Answer from the drawing. Dimensions are ordinates in mm from the lowest x, y and z of the part. A direction names the side the tool comes from. Coordinates: 2 decimals unless noted, no trailing zeros. Write each loop counter-clockwise with the first axis right and the second up, starting at its lowest first coordinate (ties: lowest second). Pieces come first, ordered by that corner, then holes. Notation, with made-up numbers: (31, -20) -> (86, -20) arc R10 ccw to (86, -12) -> close; hole circle Ø4 at (44.25, 73). An arc over 180 degrees is marked (long way). One line per item, written item: value. Start each with the question number.
1. Consider line 1 along Y through (x, z) = (15, 23.75); line 2 along X through (y, z) = (2.5, 14.5); line 3 along Y through (x, z) = (19, 14.25). Determine where each line is inside the solid, lowest interval first.
2. Given P1, Ø3, axis at x = 4.5, y = 7.5, coming from the +Z side; P2, Ø12, axis at y = 3, z = 9, coming from the +X side; P3, Ø3, axis at x = 20, y = 6.5, coming from the +Z side; P4, Ø3, axis at y = 18, z = 13.5, coming from the +X side, each flat-ended and moving along its own axis, determine where each tip first touches the part or whether it passes through.
3. Find section D-D, the plane y = 16.25. Write down the section's boundary in (x, z).
4. For the marked faces 1, 2 and 3, determine the directions among +Z, -Z, +X, -X, +Y, -Y from which every point of the face is accessible in a straight line to the end or side of a thin tool.
5. Find section C-C, the plane y = 4.25. Write down the section's boundary in (x, z), and give its area (3 significant figures).
6. Find section A-A, the plane z = 15. Write down the section's boundary in (x, y).
7. Find section B-B, the plane x = 15. Write down the section's boundary in (y, z).
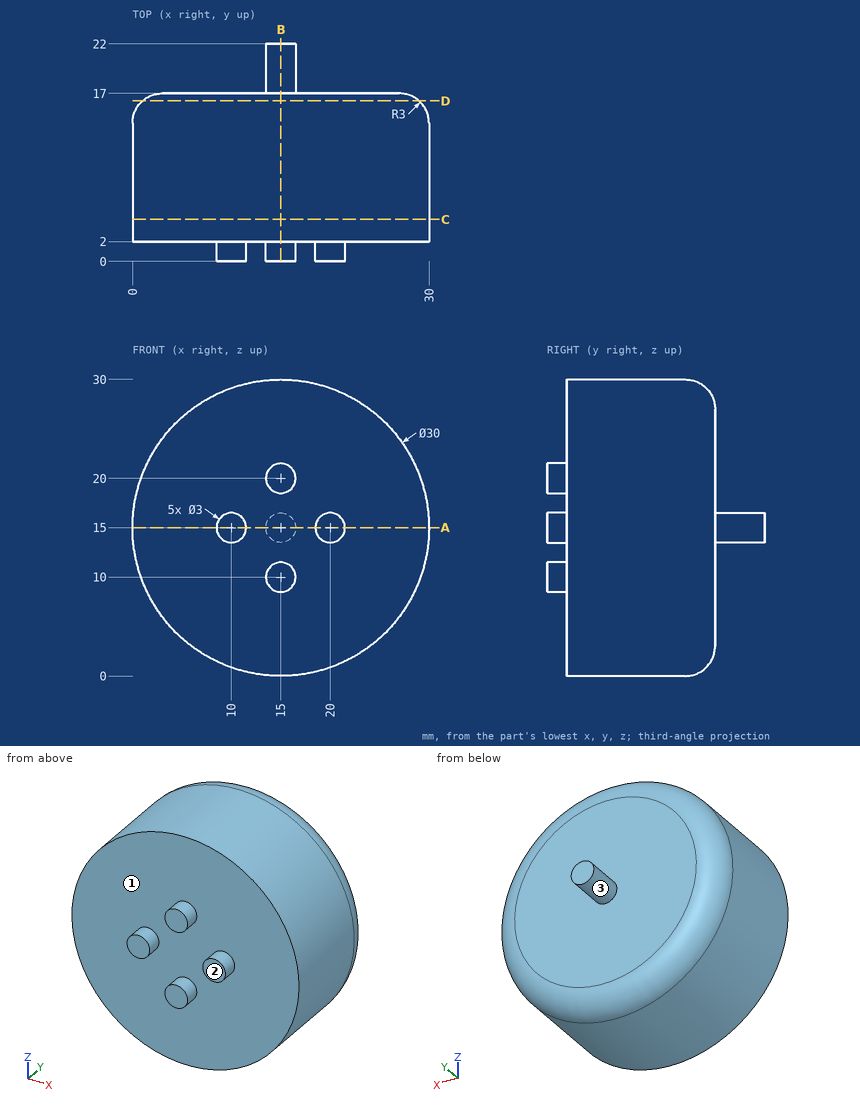
Answer block:
1. line 1: y = 2 to 17
1. line 2: x = 0.01 to 29.99
1. line 3: y = 0 to 17
2. P1: stops at z = 27
2. P2: stops at x = 30
2. P3: stops at z = 29.59
2. P4: stops at x = 28.58
3. outline: circle Ø27.97 at (15, 15)
4. face 1: -Y
4. face 2: +Z, -Z, +X, -X, -Y
4. face 3: +Y
5. outline: circle Ø30 at (15, 15)
5. area: 707 mm2
6. outline: (0, 2) -> (8.5, 2) -> (8.5, 0) -> (11.5, 0) -> (11.5, 2) -> (18.5, 2) -> (18.5, 0) -> (21.5, 0) -> (21.5, 2) -> (30, 2) -> (30, 14) arc R3 ccw to (27, 17) -> (16.5, 17) -> (16.5, 22) -> (13.5, 22) -> (13.5, 17) -> (3, 17) arc R3 ccw to (0, 14) -> close
7. outline: (0, 8.5) -> (2, 8.5) -> (2, 0) -> (14, 0) arc R3 ccw to (17, 3) -> (17, 13.5) -> (22, 13.5) -> (22, 16.5) -> (17, 16.5) -> (17, 27) arc R3 ccw to (14, 30) -> (2, 30) -> (2, 21.5) -> (0, 21.5) -> (0, 18.5) -> (2, 18.5) -> (2, 11.5) -> (0, 11.5) -> close
